Model file for the job. Use its own axes, mm. A direction names the side the tool comes from. Round coordinates to 2 decimals unless told otherwise and drop trailing zeros. Loops run counter-clockwise (first coordinate to the right, second up) from the corner with the lowest first, then second, coordinate; pieces in that order, holes last. Notation, with made-up numbers: (59.5, 12.5) -> (111.5, 12.5) arc R14 cw to (111.5, 26.5) -> close; hole circle Ø11 at (48.5, 21.25). An arc over 180 degrees is marked (long way). Use a Markdown table: item, result.
from build123d import *

# Parameters (mm, degrees)
EXTRUDE_1_DEPTH      = 3
EXTRUDE_1_DEPTH_BACK = 1
SKETCH_2_R           = 4.5
SKETCH_2_R_2         = 3
EXTRUDE_2_DEPTH      = 20
SKETCH_3_R           = 3
CUT_EXTRUDE_1_DEPTH  = 34.900589965
CUT_EXTRUDE_2_REACH  = 35.901
SKETCH_4_R           = 9.774013962
SKETCH_5_W           = 13.881504323
SKETCH_5_H           = 4
CUT_EXTRUDE_4_DEPTH  = 34.900589965


with BuildPart() as part:
    # Эскиз1 → Бобышка-Вытянуть1 (new, two sides: drawn at the far end of the back side and taken through both)
    with BuildSketch(Plane.XY.offset(-EXTRUDE_1_DEPTH_BACK)):
        with BuildLine():
            Line((23.759671021, 9.680123705), (0, 18.61347829))
            Line((0, 18.61347829), (0, 7.93))
            Line((0, 7.93), (20.240328979, 0.319876295))
            ThreePointArc((20.240328979, 0.319876295), (26.680123705, 3.240328979), (23.759671021, 9.680123705))
        make_face()
        with BuildLine():
            Line((8.951842855, 7.235082801), (21.12016449, 2.659938147))
            ThreePointArc((21.12016449, 2.659938147), (24.340061853, 4.12016449), (22.87983551, 7.340061853))
            Line((22.87983551, 7.340061853), (10.711513876, 11.915206507))
            ThreePointArc((10.711513876, 11.915206507), (7.491616513, 10.454980164), (8.951842855, 7.235082801))
        make_face(mode=Mode.SUBTRACT)
    extrude(amount=EXTRUDE_1_DEPTH + EXTRUDE_1_DEPTH_BACK)

    # Эскиз2 → Бобышка-Вытянуть2 (add)
    with BuildSketch(Plane(origin=(0, 0, 0), x_dir=(1, 0, 0), z_dir=(0, 1, 0))):
        with Locations(Location((0, 0, 0), (0, 0, 270))):
            Circle(SKETCH_2_R)
        with Locations(Location((0, 0, 0), (0, 0, 270))):
            Circle(SKETCH_2_R_2, mode=Mode.SUBTRACT)
    extrude(amount=EXTRUDE_2_DEPTH)

    # Эскиз3 → Вырез-Вытянуть1 (cut, through all)
    with BuildSketch(Plane(origin=(0, 0, 0), x_dir=(-1, 0, 0), z_dir=(0, -1, 0))):
        with Locations(Location((0, 0, 0), (0, 0, 270))):
            Circle(SKETCH_3_R)
    extrude(amount=-CUT_EXTRUDE_1_DEPTH, mode=Mode.SUBTRACT)

    # Вырез-Вытянуть2: up to this face of the body (flat: up to its plane)
    cut_extrude_2_end = Plane(part.part.faces().sort_by_distance((12.227229865, 3.33270655, 1.020399835))[0])
    # Эскиз4 → Вырез-Вытянуть2 (cut, up to the picked face)
    with BuildSketch(Plane.XZ, mode=Mode.PRIVATE) as cut_extrude_2_sk1:
        Circle(SKETCH_4_R)
    cut_extrude_2_tool1 = split(extrude(cut_extrude_2_sk1.sketch, amount=-CUT_EXTRUDE_2_REACH, mode=Mode.PRIVATE), bisect_by=cut_extrude_2_end, keep=Keep.BOTH, mode=Mode.PRIVATE)
    add(cut_extrude_2_tool1.solids().sort_by(Axis((0, 0, 0), (0, 1, 0)))[0], mode=Mode.SUBTRACT)

    # Эскиз5 → Вырез-Вытянуть4 (cut, through all)
    with BuildSketch(Plane(origin=(0, 0, 0), x_dir=(1, 0, 0), z_dir=(0, 1, 0))):
        with Locations((-7.880628676, 0)):
            Rectangle(SKETCH_5_W, SKETCH_5_H)
    extrude(amount=CUT_EXTRUDE_4_DEPTH, mode=Mode.SUBTRACT)


solid = part.part
Q1. Band-saw the part on B-B, the plane y = 5. Give the cut face in (x, z), plus the area to 3 significant figures.
Results list:
| item | result |
|---|---|
| outline | (7.79, -1) -> (14.9, -1) -> (14.9, 3) -> (7.79, 3) -> close; (24.5, -1) -> (27, -1) -> (27, 3) -> (24.5, 3) -> close |
| area | 38.4 mm² |
Q2. Tool access for faces 4 (the face through (-3, 14, -2)), 5 (the face through (14.95, 4.98, 0.97)), 6 (the face through (15, 11, 3)): list every direction of +Z, -Z, +X, -X, +Y, -Y with a clear straight run to the whole face (end or side of a thin tool).
Results list:
| item | result |
|---|---|
| face 4 | -X, +Y, -Y |
| face 5 | +Z, -Z |
| face 6 | +Z, +X, +Y, -Y |
Q3. Drill centre lines: L1, parallel to Z at x = 0, y = 10.25; L2, parallel to Z at x = 20, y = 3; L3, parallel to Y at x = 21.5, z = 0.5. Where is each one in solid material? Low to high. Write a range as from..to.
Results list:
| item | result |
|---|---|
| L1 | z = -4.5..-3, 3..4.5 |
| L2 | z = -1..3 |
| L3 | y = 0.03..2.55, 7.86..10.53 |
Q4. Band-saw the part on C-C, the plane z = 0. Give the cut face in (x, y), plus the area to 3 significant figures.
Results list:
| item | result |
|---|---|
| outline | (3, 6.8) -> (20.24, 0.32) arc R5 ccw to (23.76, 9.68) -> (4.5, 16.92) -> (4.5, 20) -> (3, 20) -> close; hole (8.95, 7.24) -> (21.12, 2.66) arc R2.5 ccw to (22.88, 7.34) -> (10.71, 11.92) arc R2.5 ccw to start |
| area | 162 mm² |
Q5. Band-saw the part on D-D, the plane y = 18.25. Give the cut face in (x, z).
Results list:
| item | result |
|---|---|
| outline | (-4.03, -2) arc R4.5 ccw (long way) to (-4.03, 2) -> (-2.24, 2) arc R3 cw (long way) to (-2.24, -2) -> close |
Q6. Pull direction Y, two halves, no side cores. Call faces 1 (the face through (13.7, 13.463, 0.972)), 2 (the face through (7.512, 10.506, 0.972)), 3 (the face through (15.6, 10.4, -1)): released by +Y, released by -Y, zero draft, split by the parting line, or undercut.
Results list:
| item | result |
|---|---|
| face 1 | released by +Y |
| face 2 | undercut |
| face 3 | zero draft |
Q7. Band-saw the part on A-A, the plane x = 0. Give the cut face in (y, z).
Results list:
| item | result |
|---|---|
| outline | (7.93, -4.5) -> (20, -4.5) -> (20, -3) -> (7.93, -3) -> close; (7.93, 3) -> (20, 3) -> (20, 4.5) -> (7.93, 4.5) -> close |
Q8. Flat gauge pins, fed straight in: pin 1 (3 mm diameter, centred on x = 22, y = 6.5, fed in from -Z); pin 2 (5 mm diameter, centred on x = 15, y = 5.5, fed in from +Z); pin 3 (5 mm diameter, centred on y = 9.5, z = 1, fed in from +X). Where does each tip first touch, or does it go through?
Results list:
| item | result |
|---|---|
| pin 1 | stops at z = -1 |
| pin 2 | stops at z = 3 |
| pin 3 | stops at x = 26.58 |
